Autodesk Inventor part; units mm, degrees
ref_plane "YZ Plane" through (0, 0, 0) normal (1, 0, 0) x (0, 1, 0)
ref_plane "XZ Plane" through (0, 0, 0) normal (0, 1, 0) x (-1, 0, 0)
ref_plane "XY Plane" through (0, 0, 0) normal (0, 0, 1) x (1, 0, 0)
sketch "Szkic1" plane through (0, 0, 0) normal (0, 1, 0) x (-1, 0, 0)
  circle A0 centre (0, 0) radius 23 construction
  arc A1 (0, 23) -> (0, -23) centre (0, 0) ccw
  line L0 (0, 23) -> (0, 27.5)
  line L1 (0, -23) -> (0, -27.5)
  line L2 (0, -38.5) -> (0, 38.5)
  arc A2 (0, 27.5) -> (0, -27.5) centre (0, 0) ccw
  line L3 (-76, 3.25) -> (-27.3073, 3.25)
  line L4 (-27.3073, 3.25) -> (-27.3073, -3.25) construction
  line L5 (-27.3073, -3.25) -> (-76, -3.25)
  line L6 (-76, -3.25) -> (-76, 3.25)
  line L7 (42.8, 0) -> (-95.8, 0)
  circle A3 centre (-66, 0) radius 1.75
  circle A4 centre (-56, 0) radius 1.75
  point P0 (-27.5, 0)
  point P1 (-23, 0)
  dimension "d0" = 46
  dimension "d1" = 4.5
  dimension "d2" = 4.5
  dimension "d3" = 6.5
  dimension "d4" = 76
  dimension "d5" = 3.5
  dimension "d6" = 10
  dimension "d7" = 10
extrude "Wyciągnięcie proste1" add sketch "Szkic1" along normal blind 6.5 contours A1 L7 A2 L0 | A1 L1 A2 L7 | L7 A4 A3 L6 L3 A2 | A2 L5 L6 L7 A3 A4
sketch "Szkic2" plane through (76, 0, -3.25) normal (0, 0, -1) x (-1, 0, 0)
  line L0 (0, 0) -> (48.6927, 0)
  line L1 (48.6927, 0) -> (48.6927, 6.5)
  line L2 (0, 6.5) -> (48.6927, 6.5)
  line L3 (0, 0) -> (0, 6.5)
  line L4 (48.6927, 0) -> (48.6927, 6.5)
  line L5 (48.6927, 3.25) -> (0, 3.25) construction
  circle A0 centre (15, 3.25) radius 1.75
  circle A1 centre (25, 3.25) radius 1.75
  point P0 (76, 0)
  dimension "d10" = 3.5
  dimension "d11" = 3.5
  dimension "d12" = 15
  dimension "d13" = 10
extrude "Wyciągnięcie proste2" cut sketch "Szkic2" against normal up to surface (6.5 mm away) contours A0 | A1
fillet "Zaokrąglenie1" radius 5 2 edges at (27.3073, 3.25, 3.25) (27.3073, 3.25, -3.25)
fillet "Zaokrąglenie2" radius 1.2 6 edges at (0, 3.25, 27.5) (0, 3.25, 23) (0, 3.25, -23) (0, 3.25, -27.5) (76, 3.25, 3.25) (76, 3.25, -3.25)
equation "\"d8\" = d3"
equation "\"d14\" = d3"
properties part number "stojak"
Source: CAD feature listing. Evaluate the final solid. Frame: model axes, mm. A direction names the side the tool comes from. Round coordinates to 2 decimals unless told otherwise and drop trailing zeros. Loops run counter-clockwise (first coordinate to the right, second up) from the corner with the lowest first, then second, coordinate; pieces in that order, holes last. Notation, with made-up numbers: (43, 23.5) - (48, 23.5) arc R20 ccw to (48, 35.5) - close; hole circle Ø8 at (76, -0.75). An arc over 180 degrees is marked (long way). Write item = value, one per line. Start each with the question number.
(1) Pin query (flat end, axial travel): pin 1 (1 mm diameter, centred on x = 66, y = 3.5, fed in from -Z); pin 2 (1 mm diameter, centred on x = 11.5, y = 5.5, fed in from -Z); pin 3 (1.5 mm diameter, centred on y = 1, z = 7.5, fed in from -X). Return the tip coordinate at first contact, or that it passes through.
(2) Section query B-B, the plane z = 0. Output: boundary loops of the cut face in (x, y), plus the area to 3 significant figures.
(3) Set-up query: faces 1 (the face through (53, 3, -3.25)), 2 (the face through (54.383, 3.204, 0.67)), 3 (the face through (53, 3, 3.25)). Return all of +Z, -Z, +X, -X, +Y, -Y with unobstructed straight access to the full face (end or side cutting, diameter ignored); none if empty.
(4) Pull-direction query (X, two-part tool) for faces 4 (the face through (0, 3, -25)), 5 (the face through (28.345, 3.296, -4.319)), 6 (the face through (59.383, 2.58, -0.046)), 7 (the face through (33, 6.5, 0)); classes: +X half, -X half, draft (parallel to the pull), parting line (faces both ways), or undercut.
(5) Section query D-D, the plane x = 8.5. Output: boundary loops of the cut face in (y, z), plus the area to 3 significant figures.
(6) Section query C-C, the plane x = 61. Output: boundary loops of the cut face in (y, z).
(7) Ray query, line 1 along Y through (x, z) = (61, -1.25); line 2 along Z through (x, y) = (66, 3.5); line 3 along X through (y, z) = (3.75, 0). Return the intervals inside material, ascending. Write a range as from..to.
(8) Section query A-A, the plane y = 3.25. Output: boundary loops of the cut face in (x, z), plus the area to 3 significant figures.
Conclusion:
q1.pin_1 = -3.25
q1.pin_2 = -25.2
q1.pin_3 = 21.47
q2.outline = (23, 0) - (54.25, 0) - (54.25, 6.5) - (23, 6.5) - close; (57.75, 0) - (64.25, 0) - (64.25, 6.5) - (57.75, 6.5) - close; (67.75, 0) - (76, 0) - (76, 6.5) - (67.75, 6.5) - close; hole circle Ø3.5 at (51, 3.25); hole circle Ø3.5 at (61, 3.25)
q2.area = 280 mm2
q3.face_1 = -Z, +X, +Y, -Y
q3.face_2 = +Y, -Y
q3.face_3 = +Z, +X, +Y, -Y
q4.face_4 = -X half
q4.face_5 = +X half
q4.face_6 = undercut
q4.face_7 = draft
q5.outline = (0, -26.15) - (6.5, -26.15) - (6.5, -21.37) - (0, -21.37) - close; (0, 21.37) - (6.5, 21.37) - (6.5, 26.15) - (0, 26.15) - close
q5.area = 62.2 mm2
q6.outline = (0, -3.25) - (1.5, -3.25) - (1.5, 3.25) - (0, 3.25) - close; (5, -3.25) - (6.5, -3.25) - (6.5, 3.25) - (5, 3.25) - close
q7.line_1 = 0..1.5, 5..6.5
q7.line_2 = -3.25..-1.75, 1.75..3.25
q7.line_3 = 23..49.32, 52.68..54.25, 57.75..59.32, 62.68..64.25, 67.75..76
q8.outline = (0, -26.27) arc R1.2 ccw to (1.25, -27.47) arc R27.5 ccw to (26.6, -6.98) arc R5 cw to (31.44, -3.25) - (49.25, -3.25) - (49.25, 3.25) - (31.44, 3.25) arc R5 cw to (26.6, 6.98) arc R27.5 ccw to (1.25, 27.47) arc R1.2 ccw to (0, 26.27) - (0, 24.17) arc R1.2 ccw to (1.14, 22.97) arc R23 cw to (1.14, -22.97) arc R1.2 ccw to (0, -24.17) - close; (52.75, -3.25) - (59.25, -3.25) - (59.25, 3.25) - (52.75, 3.25) - close; (62.75, -3.25) - (74.8, -3.25) arc R1.2 ccw to (76, -2.05) - (76, 2.05) arc R1.2 ccw to (74.8, 3.25) - (62.75, 3.25) - close; hole circle Ø3.5 at (56, 0); hole circle Ø3.5 at (66, 0)
q8.area = 612 mm2
